Part model, mm, in its own coordinate system. Face numbers are marked on the shaded views. A direction names the side the tool comes from. Give positions to 0.01 mm unless a question says otherwise; leave off trailing zeros. Order: outer loops, then holes, each group sorted by start corner. A loop starts at its lowest first (then second) coordinate and runs counter-clockwise, first axis right, second up. Notation, with made-up numbers: M -12.5,-17.5 L 19.5,-17.5 A33 cw 19.5,18.5 Z; hole C 59,73.5 d4. An arc over 180 degrees is marked long. One line per question, with ' | ' between items.
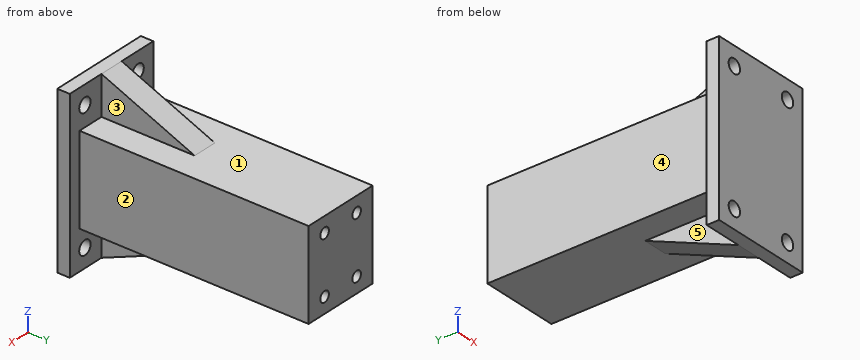
```python
from build123d import *

# Parameters (mm, degrees)
SKETCH10_W          = 33.1
SKETCH10_H          = 53.5
BOSS_EXTRUDE7_DEPTH = 4
SKETCH12_R          = 2.25
CUT_EXTRUDE2_DEPTH  = 32.709068104
SKETCH11_W          = 25.4
SKETCH11_H          = 28.5
BOSS_EXTRUDE8_DEPTH = 73.7
RIB3_REACH          = 82.132
SKETCH13_WALL_W     = 194.764219338
SKETCH13_WALL_H     = 8
SKETCH14_R          = 1.7
CUT_EXTRUDE3_DEPTH  = 12
CUT_EXTRUDE5_START  = -5
SKETCH14_3_R        = 1.7
CUT_EXTRUDE5_DEPTH  = 2.5


with BuildPart() as part:
    # Sketch10 → Boss-Extrude7 (new body)
    with BuildSketch(Plane(origin=(0, 0, 0), x_dir=(1, 0, 0), z_dir=(0, 1, 0))):
        Rectangle(SKETCH10_W, SKETCH10_H)
    extrude(amount=-BOSS_EXTRUDE7_DEPTH)

    # Sketch12 → Cut-Extrude2 (cut, through all)
    with BuildSketch(Plane(origin=(0, 0, 0), x_dir=(1, 0, 0), z_dir=(0, 1, 0))):
        with Locations(Location((-10.55, 20.75, 0), (0, 0, 270))):
            Circle(SKETCH12_R)
        with Locations(Location((10.55, 20.75, 0), (0, 0, 270))):
            Circle(SKETCH12_R)
        with Locations(Location((10.55, -20.75, 0), (0, 0, 270))):
            Circle(SKETCH12_R)
        with Locations(Location((-10.55, -20.75, 0), (0, 0, 270))):
            Circle(SKETCH12_R)
    extrude(amount=-CUT_EXTRUDE2_DEPTH, mode=Mode.SUBTRACT)

    # Sketch11 → Boss-Extrude8 (add)
    with BuildSketch(Plane(origin=(0, 0, 0), x_dir=(1, 0, 0), z_dir=(0, 1, 0))):
        Rectangle(SKETCH11_W, SKETCH11_H)
    extrude(amount=BOSS_EXTRUDE8_DEPTH)

    # Sketch13 wall → Rib3 (add, up to next)
    with BuildSketch(Plane(origin=(0, 15, -20.5), x_dir=(0, 0.923076923077, 0.384615384615), z_dir=(0, -0.384615384615, 0.923076923077)), mode=Mode.PRIVATE) as rib3_sk1:
        Rectangle(SKETCH13_WALL_W, SKETCH13_WALL_H)
    rib3_tool1 = extrude(rib3_sk1.sketch, amount=RIB3_REACH, mode=Mode.PRIVATE) - part.part
    rib3 = rib3_tool1.solids().sort_by_distance((0, 15, -20.5))[0]
    add(rib3)

    # Mirror1: Rib3 across plane
    add(rib3.mirror(Plane.XY))

    # Sketch14 → Cut-Extrude3 (cut)
    with BuildSketch(Plane(origin=(0, 73.7, 0), x_dir=(1, 0, 0), z_dir=(0, 1, 0))):
        with Locations(Location((-6.35, 9.25, 0), (0, 0, 270))):
            Circle(SKETCH14_R)
        with Locations(Location((6.35, 9.25, 0), (0, 0, 270))):
            Circle(SKETCH14_R)
        with Locations(Location((-6.35, -9.25, 0), (0, 0, 270))):
            Circle(SKETCH14_R)
        with Locations(Location((6.35, -9.25, 0), (0, 0, 270))):
            Circle(SKETCH14_R)
    extrude(amount=-CUT_EXTRUDE3_DEPTH, mode=Mode.SUBTRACT)

    # Sketch14<3> → Cut-Extrude5 (cut)
    with BuildSketch(Plane(origin=(0, 73.7, 0), x_dir=(1, 0, 0), z_dir=(0, 1, 0)).offset(CUT_EXTRUDE5_START)):
        Polygon((-2.943633412, 9.25), (-4.646816706, 12.2), (-8.053183294, 12.2), (-9.756366588, 9.25), (-8.053183294, 6.3), (-4.646816706, 6.3), align=None)
        with Locations(Location((-6.35, 9.25, 0), (0, 0, 270))):
            Circle(SKETCH14_3_R, mode=Mode.SUBTRACT)
        Polygon((9.756366588, 9.25), (8.053183294, 12.2), (4.646816706, 12.2), (2.943633412, 9.25), (4.646816706, 6.3), (8.053183294, 6.3), align=None)
        with Locations(Location((6.35, 9.25, 0), (0, 0, 270))):
            Circle(SKETCH14_3_R, mode=Mode.SUBTRACT)
        Polygon((9.756366588, -9.25), (8.053183294, -6.3), (4.646816706, -6.3), (2.943633412, -9.25), (4.646816706, -12.2), (8.053183294, -12.2), align=None)
        with Locations(Location((6.35, -9.25, 0), (0, 0, 270))):
            Circle(SKETCH14_3_R, mode=Mode.SUBTRACT)
        Polygon((-2.943633412, -9.25), (-4.646816706, -6.3), (-8.053183294, -6.3), (-9.756366588, -9.25), (-8.053183294, -12.2), (-4.646816706, -12.2), align=None)
        with Locations(Location((-6.35, -9.25, 0), (0, 0, 270))):
            Circle(SKETCH14_3_R, mode=Mode.SUBTRACT)
    extrude(amount=-CUT_EXTRUDE5_DEPTH, mode=Mode.SUBTRACT)


solid = part.part
```
1. Drop flat-ended pins along their axis: pin 1 (0.8 mm diameter, centred on x = -5.5, y = 67.5, fed in from -Z); pin 2 (2 mm diameter, centred on x = -6.35, z = -9.25, fed in from +Y); pin 3 (2 mm diameter, centred on y = 7, z = -11.5, fed in from +X); pin 4 (7 mm diameter, centred on x = 10.55, z = -20.75, fed in from -Y). Give the stop position or say it passes through.
Worked out:
pin 1: stops at z = -14.25 | pin 2: stops at y = 61.7 | pin 3: stops at x = 12.7 | pin 4: stops at y = -4
2. Slice it at D-D on z = -2. Give the cut face in (x, y), then the cut area to 3 significant figures.
Worked out:
outline: M -16.55,-4 L 16.55,-4 L 16.55,0 L 12.7,0 L 12.7,73.7 L -12.7,73.7 L -12.7,0 L -16.55,0 Z | area: 2,000 mm2
3. Tool access for the marked faces 1, 2, 3, 4 and 5: list every direction of +Z, -Z, +X, -X, +Y, -Y with a clear straight run to the whole face (end or side of a thin tool).
Worked out:
face 1: +Z, +Y | face 2: +Z, -Z, +X, +Y | face 3: +Z, +X, +Y | face 4: +Z, -Z, -X, +Y | face 5: -Z, -X, +Y
4. Slice it at A-A on z = -20.75. Give the cut face in (x, y), then the cut area to 3 significant figures.
Worked out:
outline: M -16.55,-4 L -12.8,-4 L -12.8,0 L -16.55,0 Z; M -8.3,-4 L 8.3,-4 L 8.3,0 L 4,0 L 4,14.4 L -4,14.4 L -4,0 L -8.3,0 Z; M 12.8,-4 L 16.55,-4 L 16.55,0 L 12.8,0 Z | area: 212 mm2
5. Probe L1, parallel to X at y = 69, z = 9; L2, parallel to Z at x = -6, y = 71; L3, parallel to Y at x = 8.5, z = -17. List the from-to ranges inside material, lowest first. Write a range as from..to.
Worked out:
L1: x = -12.7..-8.03, -4.67..4.67, 8.03..12.7 | L2: z = -14.25..-10.91, -7.59..7.59, 10.91..14.25 | L3: y = -4..0
6. Slice it at B-B on y = 62.5. Give the cut face in (x, z), then the cut area to 3 significant figures.
Worked out:
outline: M -12.7,-14.25 L 12.7,-14.25 L 12.7,14.25 L -12.7,14.25 Z; hole C -6.35,-9.25 d3.4; hole C -6.35,9.25 d3.4; hole C 6.35,-9.25 d3.4; hole C 6.35,9.25 d3.4 | area: 688 mm2
